The figure shows three views and two pictorial views of one solid part (mm, origin at its lowest corner). Answer the questions. A direction names the side the tool comes from. Coordinates: 2 decimals unless noted, no trailing zeros. Loops run counter-clockwise (first coordinate to the right, second up) from the corner with the lowest first, then second, coordinate; pieces in that order, holes last. Notation, with made-up numbers: (39, 21) -> (86, 21) arc R13 cw to (86, 46) -> close; hole circle Ø1 at (51.25, 29.25). An arc over 180 degrees is marked (long way). Use a Markdown table: item, result. Add a question column.
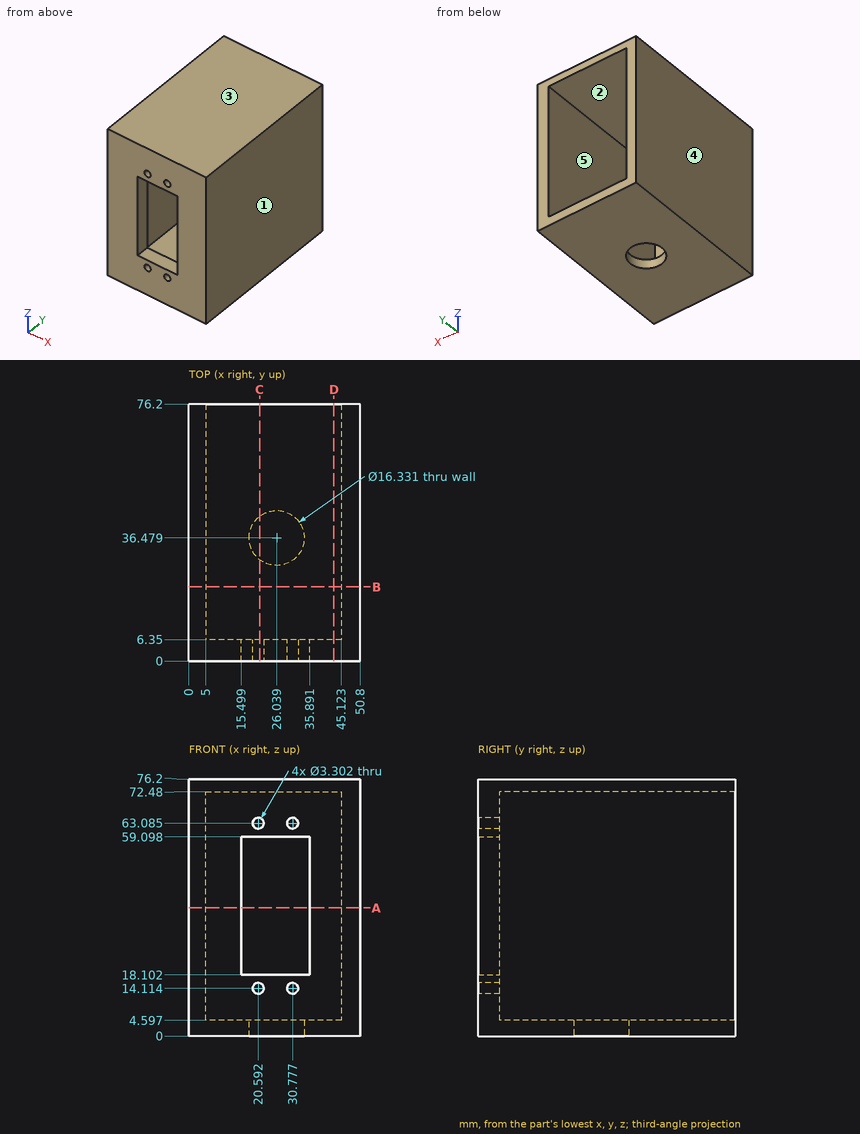
Item 1: Given pin 1 (8 mm diameter, centred on x = 11, z = 25, fed in from +Y); pin 2 (13 mm diameter, centred on x = 26.04, y = 36.48, fed in from -Z), each flat-ended and moving along its own axis, determine where each tip first touches the part or whether it passes through.
Item 2: Section B-B (y = 22) is taken. Determine the outline of the cut face in (x, z), then the cut area to 3 significant figures.
Item 3: For a pull along Z with two mould halves and no side action, classify the marked faces 1, 2 and 3 as +Z half, -Z half, draft (parallel to the pull), parting line (faces both ways), or undercut.
Item 4: For the marked faces 4 and 5, determine the directions among +Z, -Z, +X, -X, +Y, -Y from which every point of the face is accessible in a straight line to the end or side of a thin tool.
Item 5: Section C-C (x = 21) is taken. Count the separate pieces of the cut face and the enclosed holes in it.
Item 6: Section A-A (z = 38) is taken. Determine the outline of the cut face in (x, y).
Item 7: Find the intervals of material crossed by probe 1 along Z at (x, y) = (38, 40.5); probe 2 along X at (y, z) = (47.5, 34); probe 3 along Y at (x, z) = (26.5, 65.5), in increasing order.
Item 8: Section D-D (x = 43) is taken. Determine the outline of the cut face in (y, z).
Output:
| question | item | result |
|---|---|---|
| 1 | pin 1 | stops at y = 6.35 |
| 1 | pin 2 | stops at z = 72.48 |
| 2 | outline | (0, 0) -> (50.8, 0) -> (50.8, 76.2) -> (0, 76.2) -> close; hole (5, 4.6) -> (45.12, 4.6) -> (45.12, 72.48) -> (5, 72.48) -> close |
| 2 | area | 1,150 mm2 |
| 3 | face 1 | draft |
| 3 | face 2 | undercut |
| 3 | face 3 | +Z half |
| 4 | face 4 | +Z, -Z, -X, +Y, -Y |
| 4 | face 5 | +Y |
| 5 | separate pieces | 5 |
| 5 | enclosed holes | 0 |
| 6 | outline | (0, 0) -> (15.5, 0) -> (15.5, 6.35) -> (5, 6.35) -> (5, 76.2) -> (0, 76.2) -> close; (35.89, 0) -> (50.8, 0) -> (50.8, 76.2) -> (45.12, 76.2) -> (45.12, 6.35) -> (35.89, 6.35) -> close |
| 7 | probe 1 | z = 0 to 4.6, 72.48 to 76.2 |
| 7 | probe 2 | x = 0 to 5, 45.12 to 50.8 |
| 7 | probe 3 | y = 0 to 6.35 |
| 8 | outline | (0, 0) -> (76.2, 0) -> (76.2, 4.6) -> (6.35, 4.6) -> (6.35, 72.48) -> (76.2, 72.48) -> (76.2, 76.2) -> (0, 76.2) -> close |
